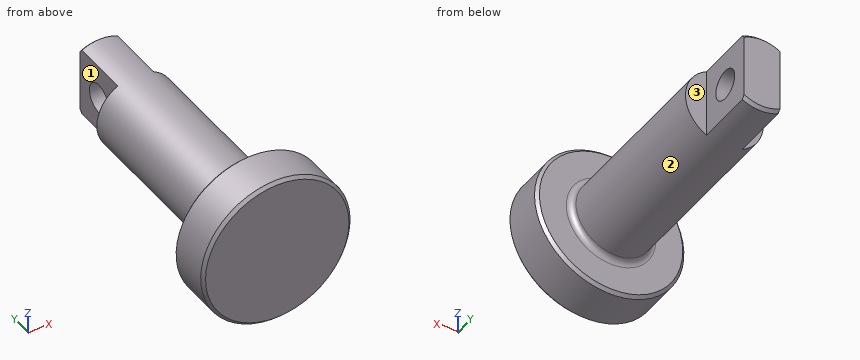
```python
from build123d import *

# Parameters (mm, degrees)
SZKIC2_R                    = 25
DODANIE_WYCI_GNI_CIE1_DEPTH = 15
SZKIC3_R                    = 13
DODANIE_WYCI_GNI_CIE2_DEPTH = 80
CHAMFER2_SIZE               = 1
CHAMFER3_SIZE               = 1
FILLET1_R                   = 2
CUT_EXTRUDE1_DEPTH          = 20
SKETCH4_R                   = 5
CUT_EXTRUDE3_DEPTH          = 12


with BuildPart() as part:
    # Szkic2 → Dodanie-wyciągnięcie1 (new body)
    with BuildSketch(Plane(origin=(0, 0, 0), x_dir=(1, 0, 0), z_dir=(0, 1, 0))):
        with Locations(Location((0, 0, 0), (0, 0, 270))):
            Circle(SZKIC2_R)
    extrude(amount=DODANIE_WYCI_GNI_CIE1_DEPTH)

    # Szkic3 → Dodanie-wyciągnięcie2 (add)
    with BuildSketch(Plane(origin=(0, 15, 0), x_dir=(1, 0, 0), z_dir=(0, 1, 0))):
        with Locations(Location((0, 0, 0), (0, 0, 270))):
            Circle(SZKIC3_R)
    extrude(amount=DODANIE_WYCI_GNI_CIE2_DEPTH)

    # Chamfer1: read off the stored shape, not the designer's step
    # Chamfer1 outline → Chamfer1 (revolve, cut)
    with BuildSketch(Plane.XY):
        Polygon((25, 15), (24, 15), (25, 14), align=None)
    revolve(axis=Axis((0, 0, 0), (0, 1, 0)), mode=Mode.SUBTRACT)

    # Chamfer2
    chamfer2_edges = [part.edges().sort_by_distance(p)[0] for p in [
        (0, 0, -25),
    ]]
    chamfer(chamfer2_edges, length=CHAMFER2_SIZE)

    # Chamfer3
    chamfer3_edges = [part.edges().sort_by_distance(p)[0] for p in [
        (0, 95, -13),
    ]]
    chamfer(chamfer3_edges, length=CHAMFER3_SIZE)

    # Fillet1
    fillet1_edges = [part.edges().sort_by_distance(p)[0] for p in [
        (0, 15, -13),
    ]]
    fillet(fillet1_edges, radius=FILLET1_R)

    # Sketch2 → Cut-Extrude1 (cut)
    with BuildSketch(Plane(origin=(0, 95, 0), x_dir=(1, 0, 0), z_dir=(0, 1, 0))):
        with BuildLine():
            Line((6, 11.993862748), (6, -11.993862748))
            ThreePointArc((6, -11.993862748), (13.41091882, 0), (6, 11.993862748))
        make_face()
        with BuildLine():
            Line((-6, -11.993862748), (-6, 11.993862748))
            ThreePointArc((-6, 11.993862748), (-13.41091882, 0), (-6, -11.993862748))
        make_face()
    extrude(amount=-CUT_EXTRUDE1_DEPTH, mode=Mode.SUBTRACT)

    # Sketch4 → Cut-Extrude3 (cut)
    with BuildSketch(Plane.ZY.offset(6)):
        with Locations((0, 85)):
            Circle(SKETCH4_R)
    extrude(amount=-CUT_EXTRUDE3_DEPTH, mode=Mode.SUBTRACT)


solid = part.part
```
CAD build for the part. Positions are in the model's coordinates, mm. Face numbers are marked on the shaded views. A direction names the side the tool comes from. Round coordinates to 2 decimals unless told otherwise and drop trailing zeros. Order: outer loops, then holes, each group sorted by start corner. A loop starts at its lowest first (then second) coordinate and runs counter-clockwise, first axis right, second up. Notation, with made-up numbers: (61, 54.5) - (73, 54.5) arc R15 cw to (73, 77.5) - close; hole circle Ø10 at (-14, 79). An arc over 180 degrees is marked (long way). Answer as CSV lines item,"result". Start each with the question number.
1. Saw through at C-C, the plane y = 58. Write the cut outline in (x, z).
2. Drill centre lines: L1, parallel to Y at x = 3, z = 0; L2, parallel to Y at x = -22, z = -3; L3, parallel to Y at x = 8, z = -10. Where is each one in solid material? Low to high. Write a range as [from, to].
3. Saw through at A-A, the plane y = 85. Write the cut outline in (x, z), and give its area (3 significant figures).
4. Pin check, flat tips, straight feed: pin 1 (22 mm diameter, centred on y = 84.5, z = -3.5, fed in from -X); pin 2 (16 mm diameter, centred on y = 85, z = 0, fed in from -X); pin 3 (3 mm diameter, centred on x = -6, y = 18.5, fed in from +Z); pin 4 (1 mm diameter, centred on x = 14, y = 24, fed in from -Z). Stop position of each tip, or through.
5. Tool access for the marked faces 1, 2 and 3: list every direction of +Z, -Z, +X, -X, +Y, -Y with a clear straight run to the whole face (end or side of a thin tool).
6. Saw through at B-B, the plane x = 0. Write the cut outline in (y, z), and give its area (3 significant figures).
Model answer:
1,outline,"circle Ø26 at (0, 0)"
2,L1,"y = [0, 80], [90, 95]"
2,L2,"y = [0, 15]"
2,L3,"y = [0, 75]"
3,outline,"(-6, -11.53) arc R13 ccw to (6, -11.53) - (6, -5) - (-6, -5) - close; (-6, 5) - (6, 5) - (6, 11.53) arc R13 ccw to (-6, 11.53) - close"
3,area,"181 mm²"
4,pin 1,"stops at x = -13"
4,pin 2,"stops at x = -6"
4,pin 3,"stops at z = 12.2"
4,pin 4,"passes through"
5,face 1,"+Z, -Z, -X, +Y"
5,face 2,"+Y"
5,face 3,"+Z, -Z, +X, +Y"
6,outline,"(0, -24) - (1, -25) - (14, -25) - (15, -24) - (15, -15) arc R2 cw to (17, -13) - (94, -13) - (95, -12) - (95, 12) - (94, 13) - (17, 13) arc R2 cw to (15, 15) - (15, 24) - (14, 25) - (1, 25) - (0, 24) - close; hole circle Ø10 at (85, 0)"
6,area,"2,750 mm²"
